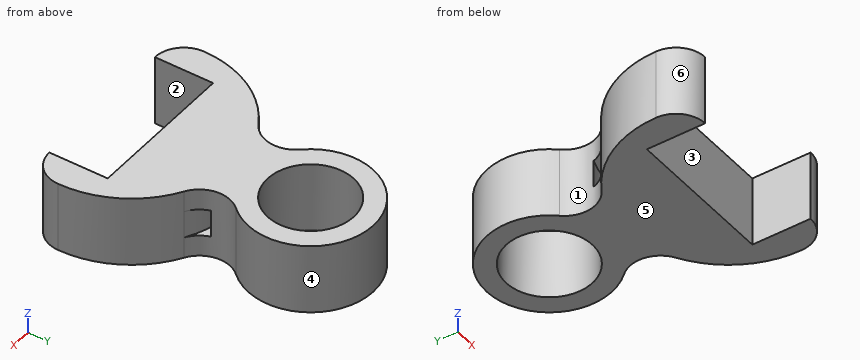
from build123d import *

# Parameters (mm, degrees)
SKETCH_R     = 8.6
PAD_DEPTH    = 7
POCKET_DEPTH = 2.75


with BuildPart() as part:
    # Sketch → Pad (new body, symmetric)
    with BuildSketch(Plane.XY):
        with BuildLine():
            ThreePointArc((9.208059, -8.4535), (0, 12.5), (-9.208059, -8.4535))
            ThreePointArc((-10.598151, -17.864192), (-7.660974, -13.49004), (-9.208059, -8.4535))
            ThreePointArc((-10.598151, -17.864192), (-18.095301, -25.509629), (-20.794271, -35.871845))
            ThreePointArc((-20.794271, -35.871845), (-19.085742, -39.948082), (-15, -41.633753))
            Line((-15, -41.633753), (-15, -30))
            Line((-15, -30), (15, -30))
            Line((15, -30), (15, -41.633753))
            ThreePointArc((15, -41.633753), (19.085742, -39.948082), (20.794271, -35.871845))
            ThreePointArc((20.794271, -35.871845), (18.095301, -25.509629), (10.598151, -17.864192))
            ThreePointArc((9.208059, -8.4535), (7.660974, -13.49004), (10.598151, -17.864192))
        make_face()
        Circle(SKETCH_R, mode=Mode.SUBTRACT)
    extrude(amount=PAD_DEPTH, both=True)

    # Sketch001 → Pocket (cut, symmetric)
    with BuildSketch(Plane.XY):
        with BuildLine():
            ThreePointArc((10.598151, -17.864192), (0, -14.960779), (-10.598151, -17.864192))
            Line((-11.617468, -16.143439), (-10.598151, -17.864192))
            ThreePointArc((11.617468, -16.143439), (0, -12.960779), (-11.617468, -16.143439))
            Line((11.617468, -16.143439), (10.598151, -17.864192))
        make_face()
    extrude(amount=POCKET_DEPTH, both=True, mode=Mode.SUBTRACT)


solid = part.part
For this review, take the finished solid that the model builds, in its own axes (mm). Face numbers are marked on the shaded views. A direction names the side the tool comes from. Round coordinates to 2 decimals unless told otherwise and drop trailing zeros. Write each loop counter-clockwise with the first axis right and the second up, starting at its lowest first coordinate (ties: lowest second). Pieces come first, ordered by that corner, then holes. Notation, with made-up numbers: (54.5, 53.5) -> (110.5, 53.5) arc R18 cw to (110.5, 79.5) -> close; hole circle Ø6 at (-13, -0.5). An arc over 180 degrees is marked (long way). Put each result on its own line as item: value.
Q1. Consider section A-A on y = 0. State the section outline as (x, z) points.
Determined:
outline: (-12.5, -7) -> (-8.6, -7) -> (-8.6, 7) -> (-12.5, 7) -> close; (8.6, -7) -> (12.5, -7) -> (12.5, 7) -> (8.6, 7) -> close
Q2. Machinability: for the marked faces 1 and 2, which of the approach directions +Z, -Z, +X, -X, +Y, -Y give a long, thin tool a straight path to every point of the face, cutting with its end or side? Answer none if there is none.
Determined:
face 1: +Z, -Z, -X
face 2: +Z, -Z, -Y
Q3. To check wall thickness, follow L1, parallel to Y at x = 0, z = 1.5; L2, parallel to Y at x = 0, z = 4; L3, parallel to X at y = -36, z = -4.75. State the ranges of each line that lie inside material, in increasing order. Write a range as [from, to].
Determined:
L1: y = [-30, -14.96], [-12.96, -8.6], [8.6, 12.5]
L2: y = [-30, -8.6], [8.6, 12.5]
L3: x = [-20.79, -15], [15, 20.79]
Q4. Consider section B-B on x = 0. State the section outline as (y, z) points.
Determined:
outline: (-30, -7) -> (-8.6, -7) -> (-8.6, 7) -> (-30, 7) -> close; (8.6, -7) -> (12.5, -7) -> (12.5, 7) -> (8.6, 7) -> close; hole (-14.96, -2.75) -> (-12.96, -2.75) -> (-12.96, 2.75) -> (-14.96, 2.75) -> close
Q5. Clearance check with flat-ended pins moving along their axes: pin 1 Ø5 at (y, z) = (-25, -4) entering from +X; pin 2 Ø1.5 at (x, y) = (-11, -7) entering from -Z; pin 3 Ø7 at (x, z) = (-1, 3) entering from -Y; pin 4 Ø2 at (y, z) = (-11.5, -2.5) entering from -X. State where each tip first meets the part, or that it passes through.
Determined:
pin 1: stops at x = 19.09
pin 2: stops at z = -7
pin 3: stops at y = -30
pin 4: stops at x = -7.96
Q6. Consider section C-C on z = 0. State the section outline as (x, y) points, and give its area (3 significant figures).
Determined:
outline: (-20.79, -35.87) arc R5.79 ccw to (-15, -41.63) -> (-15, -30) -> (15, -30) -> (15, -41.63) arc R5.79 ccw to (20.79, -35.87) arc R20.79 ccw to (10.6, -17.86) arc R20.79 ccw to (-10.6, -17.86) arc R20.79 ccw to start; (-9.21, -8.45) arc R6.12 cw to (-7.85, -14.36) arc R22.79 cw to (7.85, -14.36) arc R6.12 cw to (9.21, -8.45) arc R12.5 ccw (long way) to start; hole circle Ø17.2 at (0, 0)
area: 847 mm^2
Q7. The part is to be moulded in two halves that separate along X. For the marked faces 3, 4, 5 and 6, say which applies: released by +X, released by -X, zero draft, split by the parting line, or undercut.
Determined:
face 3: undercut
face 4: split by the parting line
face 5: zero draft
face 6: released by -X
Q8. Consider section D-D on z = 5.5. State the section outline as (x, y) points.
Determined:
outline: (-20.79, -35.87) arc R5.79 ccw to (-15, -41.63) -> (-15, -30) -> (15, -30) -> (15, -41.63) arc R5.79 ccw to (20.79, -35.87) arc R20.79 ccw to (10.6, -17.86) arc R6.12 cw to (9.21, -8.45) arc R12.5 ccw (long way) to (-9.21, -8.45) arc R6.12 cw to (-10.6, -17.86) arc R20.79 ccw to start; hole circle Ø17.2 at (0, 0)
